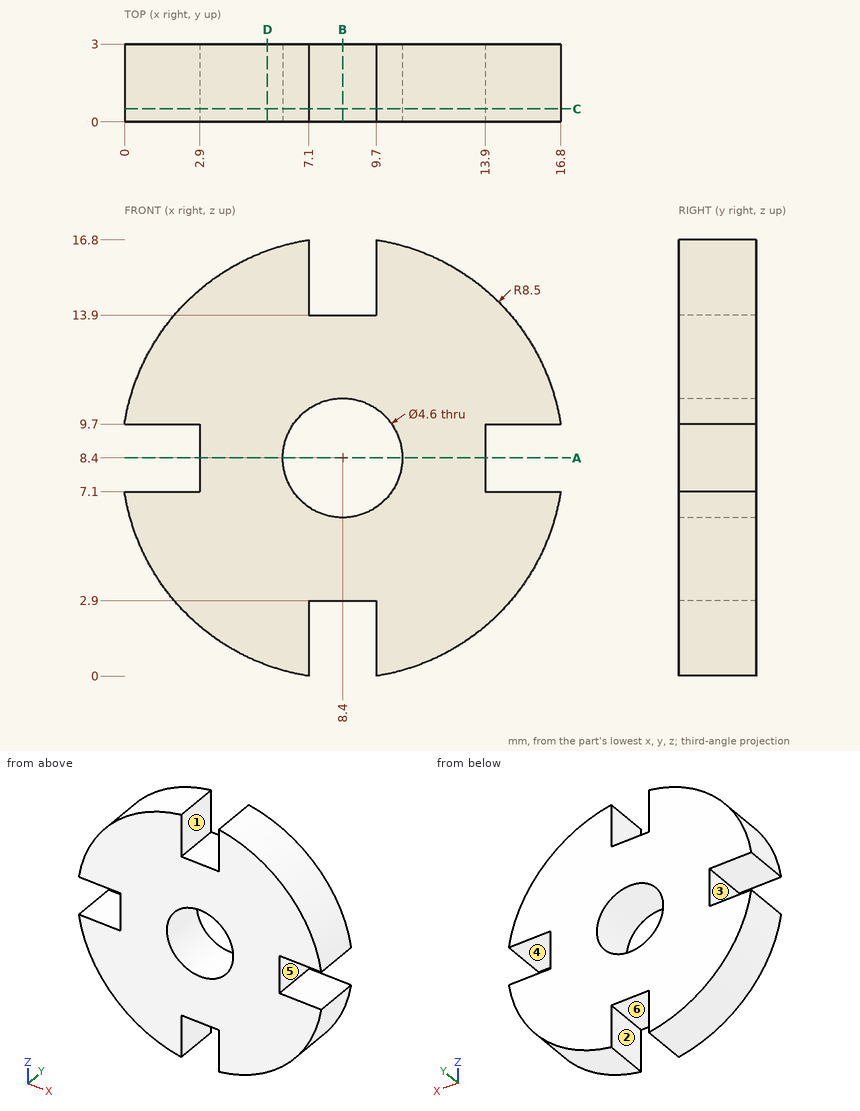
The figure shows three views and two pictorial views of one solid part (mm, origin at its lowest corner). Answer the questions. A direction names the side the tool comes from. Coordinates: 2 decimals unless noted, no trailing zeros. Loops run counter-clockwise (first coordinate to the right, second up) from the corner with the lowest first, then second, coordinate; pieces in that order, holes last. Notation, with made-up numbers: (35, 82.25) -> (82, 82.25) arc R21 cw to (82, 110.25) -> close; hole circle Ø3 at (-34, 2.5). An arc over 180 degrees is marked (long way). Use one line per item in the form item = value. Start each with the question number.
Item 1: The part is cut by section C-C on y = 0.5. Determine the outline of the cut face in (x, z).
Item 2: The part is cut by section D-D on x = 5.5. Determine the outline of the cut face in (y, z), then the cut area to 3 significant figures.
Item 3: Flat-ended cylindrical pins translate along their axes: pin 1 Ø1.5 at (y, z) = (1.5, 15.5) entering from +X; pin 2 Ø1.5 at (y, z) = (2, 1.5) entering from +X; pin 3 Ø1.5 at (x, y) = (1.5, 2) entering from -Z. Find the tip coordinate at first contact, or state that the pin passes through.
Item 4: A tool of negligible diameter and unlimited length cuts with its end or side. For the marked faces 1, 2 and 3, from which of +Z, -Z, +X, -X, +Y, -Y can it reach the whole face along a straight path? Write none if from no direction.
Item 5: The part is cut by section B-B on x = 8.4. Determine the outline of the cut face in (y, z).
Item 6: The part is cut by section A-A on z = 8.4. Determine the outline of the cut face in (x, y).
Item 7: Consider L1, parallel to X at y = 1.5, z = 8.4; L2, parallel to Z at x = 1, y = 1.95; L3, parallel to X at y = 1.8, z = 2.25. Determine where each line is inside the solid, lowest interval first. Write a range as [from, to].
Item 8: The mould has two halves that part along X. Classify the marked faces 4, 5 and 6: released by +X, released by -X, zero draft, split by the parting line, or undercut.
Answer key:
q1.outline = (0, 7.1) arc R8.5 ccw to (7.1, 0) -> (7.1, 2.9) -> (9.7, 2.9) -> (9.7, 0) arc R8.5 ccw to (16.8, 7.1) -> (13.9, 7.1) -> (13.9, 9.7) -> (16.8, 9.7) arc R8.5 ccw to (9.7, 16.8) -> (9.7, 13.9) -> (7.1, 13.9) -> (7.1, 16.8) arc R8.5 ccw to (0, 9.7) -> (2.9, 9.7) -> (2.9, 7.1) -> close; hole circle Ø4.6 at (8.4, 8.4)
q2.outline = (0, 0.41) -> (3, 0.41) -> (3, 16.39) -> (0, 16.39) -> close
q2.area = 47.9 mm2
q3.pin_1 = 14.05
q3.pin_2 = 14.27
q3.pin_3 = 2.53
q4.face_1 = +Z, +Y, -Y
q4.face_2 = -Z, +Y, -Y
q4.face_3 = -X, +Y, -Y
q5.outline = (0, 2.9) -> (3, 2.9) -> (3, 6.1) -> (0, 6.1) -> close; (0, 10.7) -> (3, 10.7) -> (3, 13.9) -> (0, 13.9) -> close
q6.outline = (2.9, 0) -> (6.1, 0) -> (6.1, 3) -> (2.9, 3) -> close; (10.7, 0) -> (13.9, 0) -> (13.9, 3) -> (10.7, 3) -> close
q7.L1 = [2.9, 6.1], [10.7, 13.9]
q7.L2 = [4.22, 7.1], [9.7, 12.58]
q7.L3 = [2.53, 7.1], [9.7, 14.27]
q8.face_4 = zero draft
q8.face_5 = released by +X
q8.face_6 = undercut
